Here's the drawing with two shaded views (mm, measured from the low corner). I have some questions. Round coordinates to 2 decimals unless told otherwise and drop trailing zeros. Order: outer loops, then holes, each group sorted by start corner. A loop starts at its lowest first (then second) coordinate and runs counter-clockwise, first axis right, second up.
Q1. If we section it at C-C (x = 157): Please give me the cut outline in (y, z).
Q2. If we section it at D-D (x = 67.5): Please give me the cut outline in (y, z), plus the area to 3 significant figures.
Q3. If we section it at B-B (z = 2.1): Please give me the cut outline in (x, y), plus the area to 3 significant figures.
Q4. Will these pins go through, and if not, where does the flat tip stop? P1, Ø1, axis at y = 39, z = 4.5, coming from the +X side; P2, Ø1.5, axis at x = 79.5, z = 1.5, coming from the +Y side; P3, Ø2.5, axis at x = 112.5, z = 2.5, coming from the -Y side; P4, Ø10, axis at x = 104.5, y = 9.5, coming from the +Z side.
Q5. If I drill on line 1 (X direction, y = 15.5, z = 1.4); line 2 (X direction, y = 13.5, z = 2.15); line 3 (Y direction, x = 157, z = 2.4), over which ranges is the centre line in solid material (lowest first)?
Q6. If we section it at A-A (x = 20): Please give me the cut outline in (y, z).
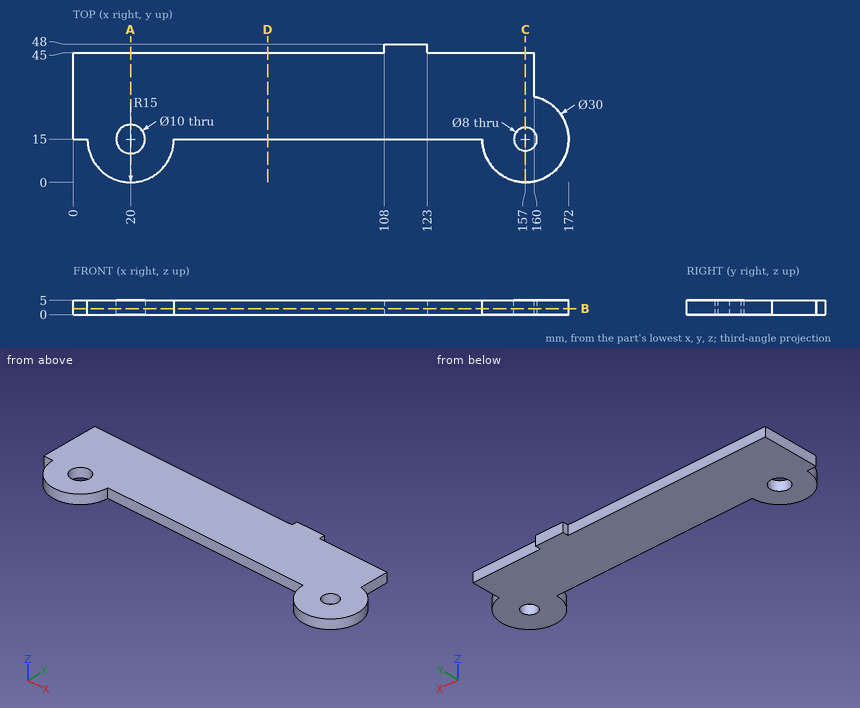
Solution:
1. outline: (0, 0) - (11, 0) - (11, 5) - (0, 5) - close; (19, 0) - (45, 0) - (45, 5) - (19, 5) - close
2. outline: (15, 0) - (45, 0) - (45, 5) - (15, 5) - close
2. area: 150 mm2
3. outline: (0, 15) - (5, 15) arc R15 ccw to (35, 15) - (142, 15) arc R15 ccw (long way) to (160, 29.7) - (160, 45) - (123, 45) - (123, 48) - (108, 48) - (108, 45) - (0, 45) - close; hole circle Ø10 at (20, 15); hole circle Ø8 at (157, 15)
3. area: 5,560 mm2
4. P1: stops at x = 160
4. P2: stops at y = 45
4. P3: stops at y = 15
4. P4: passes through
5. line 1: x = 0 to 15.03, 24.97 to 153.03, 160.97 to 171.99
5. line 2: x = 5.08 to 15.23, 24.77 to 34.92, 142.08 to 153.29, 160.71 to 171.92
5. line 3: y = 0 to 11, 19 to 45
6. outline: (0, 0) - (10, 0) - (10, 5) - (0, 5) - close; (20, 0) - (45, 0) - (45, 5) - (20, 5) - close
